Model file for the job. Use its own axes, mm. A direction names the side the tool comes from. Give positions to 0.01 mm unless a question says otherwise; leave off trailing zeros. Loops run counter-clockwise (first coordinate to the right, second up) from the corner with the lowest first, then second, coordinate; pieces in that order, holes last. Notation, with made-up numbers: M -38.5,83.25 L -33.5,83.25 A6 cw -33.5,88.25 Z; hole C 30,9.25 d7. An arc over 180 degrees is marked long. Answer in a Markdown table with one row per item.
```python
from build123d import *
from build123d import SkipClean  # not in build123d's __all__

# Parameters (mm, degrees)
F1_W      = 81.28
F1_H      = 8.128
F2_W      = 81.28
F2_H      = 8.128
F4_W      = 26.233073324
F4_H      = 20.56436991
F5_DEPTH  = 1
F6_W      = 78.105
F6_H      = 7.493
F7_W      = 78.105
F7_H      = 7.493
F9_W      = 81.28
F9_H      = 17.78
F10_DEPTH = 0.5


with BuildPart() as f3:
    # F1 (on Top) → F3 section 0
    with BuildSketch(Plane.XY):
        Rectangle(F1_W, F1_H)
    # F2 (on offset) → F3 section 1
    with BuildSketch(Plane.XY.offset(25)):
        with Locations((0, 4.064)):
            Rectangle(F2_W, F2_H)
    loft()

    # F4 (on face) → F5 (cut)
    with BuildSketch(Plane(origin=(0, -3.9593706469, 0.6436352924), x_dir=(1, 0, 0), z_dir=(0, -0.9870433569, 0.1604537681))):
        with Locations((0, 14.4417314122)):
            Rectangle(F4_W, F4_H)
    extrude(amount=-F5_DEPTH, mode=Mode.SUBTRACT)

    # F6 (on offset) → F8 section 0
    with BuildSketch(Plane.XY.offset(25)):
        with Locations((-1.3208e-06, 4.0446073394)):
            Rectangle(F6_W, F6_H)
    # F7 (on Top) → F8 section 1
    with BuildSketch(Plane.XY):
        Rectangle(F7_W, F7_H)
    loft(mode=Mode.SUBTRACT)

    # F9 (on Top) → F10 (join)
    with BuildSketch(Plane.XY):
        with Locations((-2.539e-07, 4.3180031988)):
            Rectangle(F9_W, F9_H)
    with SkipClean():  # cleaning this boolean's faces spoils the solid; the shape is the same uncleaned
        extrude(amount=-F10_DEPTH)


solid = f3.part
```
Q1. Saw through at A-A (y = 9.25). Give the cut face in (x, z), and give its area (3 significant figures).
Reported:
| item | result |
|---|---|
| outline | M -40.64,-0.5 L 40.64,-0.5 L 40.64,0 L -40.64,0 Z |
| area | 40.6 mm² |
Q2. Mould opens along X. For faces 3 (the face through (-1, 9, 0)), 4 (the face through (-1, 0, 0)) say: released by +X, released by -X, zero draft, split by the parting line, or undercut.
Reported:
| item | result |
|---|---|
| face 3 | zero draft |
| face 4 | undercut |
Q3. Probe probe 1 along X at (y, z) = (4.5, 10.5); probe 2 along Z at (x, y) = (32, 11.25); probe 3 along Y at (x, z) = (1.5, 1). List the from-to ranges inside material, lowest first.
Reported:
| item | result |
|---|---|
| probe 1 | -40.64 to -39.05, 39.05 to 40.64 |
| probe 2 | -0.5 to 0 |
| probe 3 | -3.9 to -3.58, 3.91 to 4.23 |
Q4. Drop flat-ended pins along their axis: pin 1 (2 mm diameter, centred on x = 2, z = 8.5, fed in from +Y); pin 2 (10 mm diameter, centred on x = 21.5, z = 5.5, fed in from -Y); pin 3 (12 mm diameter, centred on x = 27, z = 12, fed in from +Y); pin 4 (2.5 mm diameter, centred on x = 18.5, y = 7.5, fed in from +Z). Give the stop position or say it passes through.
Reported:
| item | result |
|---|---|
| pin 1 | y = 5.61 |
| pin 2 | y = -3.98 |
| pin 3 | y = 6.99 |
| pin 4 | z = 25 |
Q5. 3-axis set-ups, long thin cutter, end or side, ignore diameter. For faces 1 (the face through (-0.57, -3.36, 4.34)), 2 (the face through (0.569, 6.124, 12.675)): which of +Z, -Z, +X, -X, +Y, -Y reach the whole face in a straight line?
Reported:
| item | result |
|---|---|
| face 1 | +Z, +X, -X, -Y |
| face 2 | +X, -X, +Y |
